For this review, take the finished solid that the model builds, in its own axes (mm). A direction names the side the tool comes from. Give positions to 0.01 mm unless a question says otherwise; leave off trailing zeros. Order: outer loops, then holes, each group sorted by start corner. A loop starts at its lowest first (then second) coordinate and runs counter-clockwise, first axis right, second up. Notation, with made-up numbers: (77, 25) -> (86, 25) arc R21 ccw to (86, 31) -> close; hole circle Ø5 at (-4, -8). An arc over 180 degrees is marked (long way). Return JSON: item names as keys, results as strings. Group by question number.
1) Insertion check: P1, Ø1, axis at x = 15, z = 19, coming from the -Y side; P2, Ø4, axis at y = 10, z = 20, coming from the +X side; P3, Ø2, axis at x = 14, y = 24, coming from the -Z side. Each pin has a flat end and moves straight along its axis. Give the tip position at first contact, or say it passes through.
2) For faces 1 (the face through (10.16, 12, 13)), 2 (the face through (8, 24, 25.4)), list the 3-axis set-ups (+Z, -Z, +X, -X, +Y, -Y) from which the entire face can be reached by the end or side of a thin tool; tool diameter is ignored.
3) To check wall thickness, follow line 1 along Y through (x, z) = (15.24, 19.75) (3 decimals); line 2 along Y through (x, z) = (3.75, 3.75); line 3 along Y through (x, z) = (4.75, 2.5). State the ranges of each line that lie inside material, in increasing order.
4) Add section A-A (y = 30.48). Give the boundary of the cut face in (x, z) (3 decimals), then the cut area to 3 significant figures.
5) The part is to be moulded in two halves that separate along Y. For faces 3 (the face through (14.83, 28.62, 12.52)), 4 (the face through (8, 24, 0)), 5 (the face through (3.177, 7.704, 12.522)), 6 (the face through (10, 38.1, 13)), say which applies: released by +Y, released by -Y, zero draft, split by the parting line, or undercut.
6) Add section D-D (z = 5.5). Give the boundary of the cut face in (x, y) (3 decimals), then the cut area to 3 significant figures.
7) Add section B-B (x = 15.24). Give the boundary of the cut face in (y, z) (3 decimals), then the cut area to 3 significant figures.
8) Add section C-C (y = 7.62). Give the boundary of the cut face in (x, z) (3 decimals).
from build123d import *

# Parameters (mm, degrees)
SKETCH1_R           = 1.905
BOSS_EXTRUDE1_DEPTH = 25.4


with BuildPart() as part:
    # Sketch1 → Boss-Extrude1 (new body)
    with BuildSketch(Plane.XY):
        with BuildLine():
            Line((0, 0), (0, 38.1))
            Line((0, 38.1), (20.32, 38.1))
            Line((20.32, 38.1), (20.32, 25.4))
            Line((20.32, 25.4), (12.192, 25.4))
            ThreePointArc((12.192, 25.4), (10.755159021, 24.804840979), (10.16, 23.368))
            Line((10.16, 23.368), (10.16, 0))
            Line((10.16, 0), (0, 0))
        make_face()
        with Locations((5.08, 30.48)):
            Circle(SKETCH1_R, mode=Mode.SUBTRACT)
        with Locations((5.08, 7.62)):
            Circle(SKETCH1_R, mode=Mode.SUBTRACT)
        with Locations((15.24, 30.48)):
            Circle(SKETCH1_R, mode=Mode.SUBTRACT)
    extrude(amount=BOSS_EXTRUDE1_DEPTH)


solid = part.part
Evaluation:
{
 "1": {"P1": "y = 25.4", "P2": "x = 10.16", "P3": "through"},
 "2": {"face 1": "+Z, -Z, +X, -Y", "face 2": "+Z, +X, -X, +Y, -Y"},
 "3": {"line 1": "25.4 to 28.575, 32.385 to 38.1", "line 2": "0 to 6.26, 8.98 to 29.12, 31.84 to 38.1", "line 3": "0 to 5.74, 9.5 to 28.6, 32.36 to 38.1"},
 "4": {"outline": "(0, 0) -> (3.175, 0) -> (3.175, 25.4) -> (0, 25.4) -> close; (6.985, 0) -> (13.335, 0) -> (13.335, 25.4) -> (6.985, 25.4) -> close; (17.145, 0) -> (20.32, 0) -> (20.32, 25.4) -> (17.145, 25.4) -> close", "area": "323 mm^2"},
 "5": {"face 3": "undercut", "face 4": "zero draft", "face 5": "undercut", "face 6": "released by +Y"},
 "6": {"outline": "(0, 0) -> (10.16, 0) -> (10.16, 23.368) arc R2.032 cw to (12.192, 25.4) -> (20.32, 25.4) -> (20.32, 38.1) -> (0, 38.1) -> close; hole circle Ø3.81 at (5.08, 7.62); hole circle Ø3.81 at (5.08, 30.48); hole circle Ø3.81 at (15.24, 30.48)", "area": "483 mm^2"},
 "7": {"outline": "(25.4, 0) -> (28.575, 0) -> (28.575, 25.4) -> (25.4, 25.4) -> close; (32.385, 0) -> (38.1, 0) -> (38.1, 25.4) -> (32.385, 25.4) -> close", "area": "226 mm^2"},
 "8": {"outline": "(0, 0) -> (3.175, 0) -> (3.175, 25.4) -> (0, 25.4) -> close; (6.985, 0) -> (10.16, 0) -> (10.16, 25.4) -> (6.985, 25.4) -> close"}
}
